Autodesk Inventor part; units mm, degrees
ref_plane "YZ Plane" through (0, 0, 0) normal (1, 0, 0) x (0, 1, 0)
ref_plane "XZ Plane" through (0, 0, 0) normal (0, 1, 0) x (-1, 0, 0)
ref_plane "XY Plane" through (0, 0, 0) normal (0, 0, 1) x (1, 0, 0)
sketch "Sketch1" plane through (0, 0, 0) normal (0, 1, 0) x (-1, 0, 0)
  line L0 (50.8, 21.59) -> (-50.8, 21.59)
  line L1 (-50.8, 21.59) -> (-50.8, -21.59)
  line L2 (-50.8, -21.59) -> (50.8, -21.59)
  line L3 (50.8, -21.59) -> (50.8, 21.59)
  line L4 (50.8, 21.59) -> (-50.8, -21.59) construction
  line L5 (-50.8, 21.59) -> (50.8, -21.59) construction
  line L6 (60.325, 31.115) -> (-60.325, 31.115)
  line L7 (-60.325, 31.115) -> (-60.325, -31.115)
  line L8 (-60.325, -31.115) -> (60.325, -31.115)
  line L9 (60.325, -31.115) -> (60.325, 31.115)
  line L10 (60.325, 31.115) -> (-60.325, -31.115) construction
  line L11 (-60.325, 31.115) -> (60.325, -31.115) construction
  point P0 (0, 0)
extrude "Extrusion1" add sketch "Sketch1" against normal blind 9.525 contours L3 L2 L1 L0 | L9 L8 L7 L6
extrude "Extrusion2" add sketch "Sketch1" along normal blind 10.16
sketch "Sketch4" plane through (-60.325, -9.525, 31.115) normal (0, 0, 1) x (1, 0, 0)
  line L0 (0, 0) -> (0, 19.685)
  line L1 (120.65, 0) -> (0, 0)
  line L2 (0, 19.685) -> (120.65, 19.685)
  line L3 (9.525, 19.685) -> (111.125, 19.685)
  line L4 (52.2991, 19.685) -> (68.3509, 19.685)
  line L5 (0, 0) -> (120.65, 0)
  line L6 (52.2991, 0) -> (68.3509, 0)
  arc A0 (52.2991, 19.685) -> (52.2991, 0) centre (60.325, 9.8425) ccw
  arc A1 (68.3509, 0) -> (68.3509, 19.685) centre (60.325, 9.8425) ccw
  point P0 (60.325, 9.525)
  dimension "d10" = 9.8425
extrude "Extrusion4" add sketch "Sketch4" along normal blind 29.21 contours A0 L2 A1 L1
mirror "Mirror1" about plane through (0, 0, 0) normal (0, 0, 1) of "Extrusion4"
sketch "Sketch5" plane through (0, 0, 0) normal (0, 1, 0) x (1, 0, 0)
  line L0 (-50.8, 21.59) -> (-50.8, -21.59)
  line L1 (50.8, -21.59) -> (50.8, 21.59)
  point P0 (0, 0)
  point P1 (-38.1, 0)
  point P2 (38.1, 0)
  dimension "postHoleCenter" = 12.7
  dimension "d16" = 12.7
hole "Hole1" at (-38.1, 0, 0) at (38.1, 0, 0) direction (0, -1, 0) diameter 5.1054 end through all counterbore diameter 10.16 counterbore depth 2.54
equation "\"d4\" = wallThickness"
equation "\"d10\" = 0.5 * outerHeight"
equation "\"d13\" = -0.5 * outerWidth + 0.5 * overallWidth"
equation "\"wallThickness\" = 9.525"
equation "\"outerWidth\" = innerWidth + 2 * wallThickness"
equation "\"outerLength\" = innerLength + 2 * wallThickness"
equation "\"outerHeight\" = innerDepth + wallThickness"
equation "\"shortenForTestPrint\" = 76.2"
properties part number "connectorToTubeBrackets02"
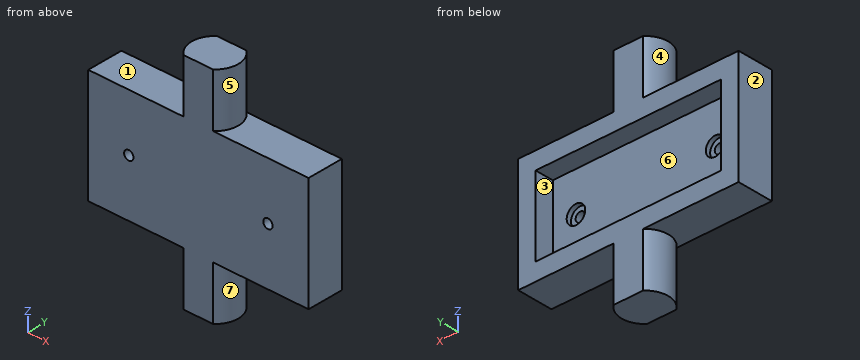
The listing builds one solid part. Answer for the finished solid, in the listing's coordinates (mm). Face numbers are marked on the shaded views. A direction names the side the tool comes from. Give positions to 0.01 mm unless a question says otherwise; leave off trailing zeros. Write each loop counter-clockwise with the first axis right and the second up, starting at its lowest first coordinate (ties: lowest second). Pieces come first, ordered by that corner, then holes. Notation, with made-up numbers: (2, 53.5) - (42, 53.5) arc R26 ccw to (42, 79.5) - close; hole circle Ø1 at (62.25, 78). An arc over 180 degrees is marked (long way). Use a Markdown table: item, result.
1. Section A-A on x = -38.1 is taken. Write down the section's boundary in (y, z) (3 decimals), plus the area to 3 significant figures.
Values follow:
| item | result |
|---|---|
| outline | (-9.525, -31.115) - (10.16, -31.115) - (10.16, -21.59) - (0, -21.59) - (0, -5.08) - (-2.54, -5.08) - (-2.54, -2.553) - (-9.525, -2.553) - close; (-9.525, 2.553) - (-2.54, 2.553) - (-2.54, 5.08) - (0, 5.08) - (0, 21.59) - (10.16, 21.59) - (10.16, 31.115) - (-9.525, 31.115) - close |
| area | 725 mm² |
2. A tool of negligible diameter and unlimited length cuts with its end or side. For the marked faces 4, 5, 6 and 7, from which of +Z, -Z, +X, -X, +Y, -Y can it reach the whole face along a straight path? Write none if from no direction.
Values follow:
| item | result |
|---|---|
| face 4 | +Z, -X |
| face 5 | +Z, +X |
| face 6 | +Y |
| face 7 | -Z, +X |
3. For a pull along Z with two mould halves and no side action, classify the marked faces 1, 2 and 3 as released by +Z, released by -Z, zero draft, split by the parting line, or undercut.
Values follow:
| item | result |
|---|---|
| face 1 | released by +Z |
| face 2 | zero draft |
| face 3 | undercut |
4. Section B-B on z = 0 is taken. Write down the section's boundary in (x, y) (3 decimals), plus the area to 3 significant figures.
Values follow:
| item | result |
|---|---|
| outline | (-60.325, -9.525) - (-40.653, -9.525) - (-40.653, -2.54) - (-43.18, -2.54) - (-43.18, 0) - (-50.8, 0) - (-50.8, 10.16) - (-60.325, 10.16) - close; (-35.547, -9.525) - (35.547, -9.525) - (35.547, -2.54) - (33.02, -2.54) - (33.02, 0) - (-33.02, 0) - (-33.02, -2.54) - (-35.547, -2.54) - close; (40.653, -9.525) - (60.325, -9.525) - (60.325, 10.16) - (50.8, 10.16) - (50.8, 0) - (43.18, 0) - (43.18, -2.54) - (40.653, -2.54) - close |
| area | 1,220 mm² |
5. Section D-D on y = -6.25 is taken. Write down the section's boundary in (x, z) (3 decimals), plus the area to 3 significant figures.
Values follow:
| item | result |
|---|---|
| outline | (-60.325, -31.115) - (-10.87, -31.115) - (-10.87, -60.325) - (10.87, -60.325) - (10.87, -31.115) - (60.325, -31.115) - (60.325, 31.115) - (10.87, 31.115) - (10.87, 60.325) - (-10.87, 60.325) - (-10.87, 31.115) - (-60.325, 31.115) - close; hole circle Ø5.105 at (-38.1, 0); hole circle Ø5.105 at (38.1, 0) |
| area | 8,740 mm² |
6. Find the intervals of material crossed by probe 1 along X at (y, z) = (-1.3, 0) (3 decimals); probe 2 along X at (y, z) = (8, 21) (3 decimals); probe 3 along Z at (x, y) = (38.1, -6.5) (3 decimals), in increasing order. Write a range as from..to.
Values follow:
| item | result |
|---|---|
| probe 1 | x = -60.325..-43.18, -33.02..33.02, 43.18..60.325 |
| probe 2 | x = -60.325..-50.8, 50.8..60.325 |
| probe 3 | z = -31.115..-2.553, 2.553..31.115 |
7. Each of these flat-tipped pins is pushed along its axis until it touches: P1, Ø10, axis at x = -41, y = 0, coming from the -Z side (3 decimals); P2, Ø16.5, axis at x = -38.1, z = 0, coming from the -Y side (3 decimals); P3, Ø16.5, axis at x = 38.1, z = 0, coming from the +Y side; P4, Ø3, axis at y = 2, z = 45, coming from the +X side. Where does it stop, or does it pass through?
Values follow:
| item | result |
|---|---|
| P1 | stops at z = -31.115 |
| P2 | stops at y = -9.525 |
| P3 | stops at y = 0 |
| P4 | stops at x = 12.7 |
8. Section C-C on y = 7.5 is taken. Write down the section's boundary in (x, z) (3 decimals).
Values follow:
| item | result |
|---|---|
| outline | (-60.325, -31.115) - (-10.474, -31.115) - (-10.474, -60.325) - (10.474, -60.325) - (10.474, -31.115) - (60.325, -31.115) - (60.325, 31.115) - (10.474, 31.115) - (10.474, 60.325) - (-10.474, 60.325) - (-10.474, 31.115) - (-60.325, 31.115) - close; hole (-50.8, -21.59) - (50.8, -21.59) - (50.8, 21.59) - (-50.8, 21.59) - close |
